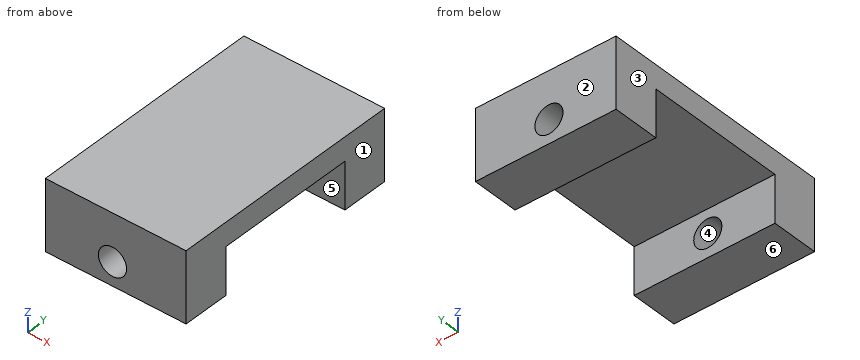
from build123d import *

# Parameters (mm, degrees)
SKETCH4_R                = 15
BOSS_EXTRUDE2_DEPTH      = 2.5
BOSS_EXTRUDE2_DEPTH_BACK = 2.5
SKETCH5_W                = 30
SKETCH5_H                = 15
SKETCH5_R                = 3
BOSS_EXTRUDE3_DEPTH      = 10


with BuildPart() as part:
    # Sketch4 → Boss-Extrude2 (new body, two sides)
    with BuildSketch(Plane.XY) as boss_extrude2_sk:
        with BuildLine():
            Line((-15, 15), (-15, -4e-09))
            ThreePointArc((-15, -4e-09), (-10.606601715, 10.606601721), (1.2e-08, 15))
            Line((1.2e-08, 15), (-15, 15))
        make_face()
        with BuildLine():
            Line((-15, -15), (0, -15))
            ThreePointArc((0, -15), (-10.606601716, -10.606601719), (-15, -4e-09))
            Line((-15, -4e-09), (-15, -15))
        make_face()
        with BuildLine():
            Line((0, -15), (15, -15))
            Line((15, -15), (15, 0))
            ThreePointArc((15, 0), (10.606601718, -10.606601718), (0, -15))
        make_face()
        Circle(SKETCH4_R)
        with BuildLine():
            ThreePointArc((1.2e-08, 15), (10.606601722, 10.606601714), (15, 0))
            Line((15, 0), (15, 15))
            Line((15, 15), (1.2e-08, 15))
        make_face()
    extrude(amount=BOSS_EXTRUDE2_DEPTH)
    extrude(boss_extrude2_sk.sketch, amount=-BOSS_EXTRUDE2_DEPTH_BACK)

    # Sketch5 → Boss-Extrude3 (add)
    with BuildSketch(Plane(origin=(0, 15, 0), x_dir=(1, 0, 0), z_dir=(0, 1, 0))):
        with Locations((0, 5)):
            Rectangle(SKETCH5_W, SKETCH5_H)
        with Locations((-0.685637394, 7.5)):
            Circle(SKETCH5_R, mode=Mode.SUBTRACT)
    boss_extrude3 = extrude(amount=BOSS_EXTRUDE3_DEPTH)

    # Mirror1: Boss-Extrude3 across plane
    add(boss_extrude3.mirror(Plane.ZX))


solid = part.part
Verification items for the finished model (mm, model axes). Face numbers are marked on the shaded views. A direction names the side the tool comes from. Coordinates: 2 decimals unless noted, no trailing zeros. Loops run counter-clockwise (first coordinate to the right, second up) from the corner with the lowest first, then second, coordinate; pieces in that order, holes last. Notation, with made-up numbers: M -10.75,14 L 23.25,14 A22 cw 23.25,41 Z; hole C -28.5,-9 d10. An arc over 180 degrees is marked long. One line per item, written item: value.
1. Section check B-B on y = 21. Record the cut outline in (x, z), plus the area to 3 significant figures.
Answers follow:
outline: M -15,-12.5 L 15,-12.5 L 15,2.5 L -15,2.5 Z; hole C -0.69,-7.5 d6
area: 422 mm^2
2. Section check C-C on z = -3. Record the cut outline in (x, y), plus the area to 3 significant figures.
Answers follow:
outline: M -15,-25 L 15,-25 L 15,-15 L -15,-15 Z; M -15,15 L 15,15 L 15,25 L -15,25 Z
area: 600 mm^2
3. Mould release check, pull along X, two halves, no side actions. Record for the marked faces 1, 2, 3 and 4: pulls with the +X half, pulls with the -X half, needs draft (parallel to the pull), parting line crosses it, or undercut.
Answers follow:
face 1: pulls with the +X half
face 2: needs draft
face 3: pulls with the -X half
face 4: undercut
4. Section check A-A on z = -7.5. Record the cut outline in (x, y).
Answers follow:
outline: M -15,-25 L -3.69,-25 L -3.69,-15 L -15,-15 Z; M -15,15 L -3.69,15 L -3.69,25 L -15,25 Z; M 2.31,-25 L 15,-25 L 15,-15 L 2.31,-15 Z; M 2.31,15 L 15,15 L 15,25 L 2.31,25 Z
5. Set-up check for the marked faces 5 and 6: record each of +Z, -Z, +X, -X, +Y, -Y from which the full face is reachable in a straight line by a thin tool's end or side.
Answers follow:
face 5: -Z, +X, -X
face 6: -Z, +X, -X, +Y, -Y
6. Section check D-D on x = 11. Record the cut outline in (y, z), plus the area to 3 significant figures.
Answers follow:
outline: M -25,-12.5 L -15,-12.5 L -15,-2.5 L 15,-2.5 L 15,-12.5 L 25,-12.5 L 25,2.5 L -25,2.5 Z
area: 450 mm^2
7. Gauge pin test, flat ends, axial feed: P1, Ø4, axis at x = -4, y = -10, coming from the -Z side; P2, Ø12, axis at x = -6.5, y = -11.5, coming from the -Z side. Record the tip position at first contact, or that the pin passes through.
Answers follow:
P1: z = -2.5
P2: z = -12.5
8. Material ranges on line 1 along X through (y, z) = (19, -7.5); line 2 along Y through (x, z) = (-4.5, -6.5); line 3 along Z through (x, y) = (-10.25, 14.5), recorded low to high. Write a range as from..to.
Answers follow:
line 1: -15..-3.69, 2.31..15
line 2: -25..-15, 15..25
line 3: -2.5..2.5
